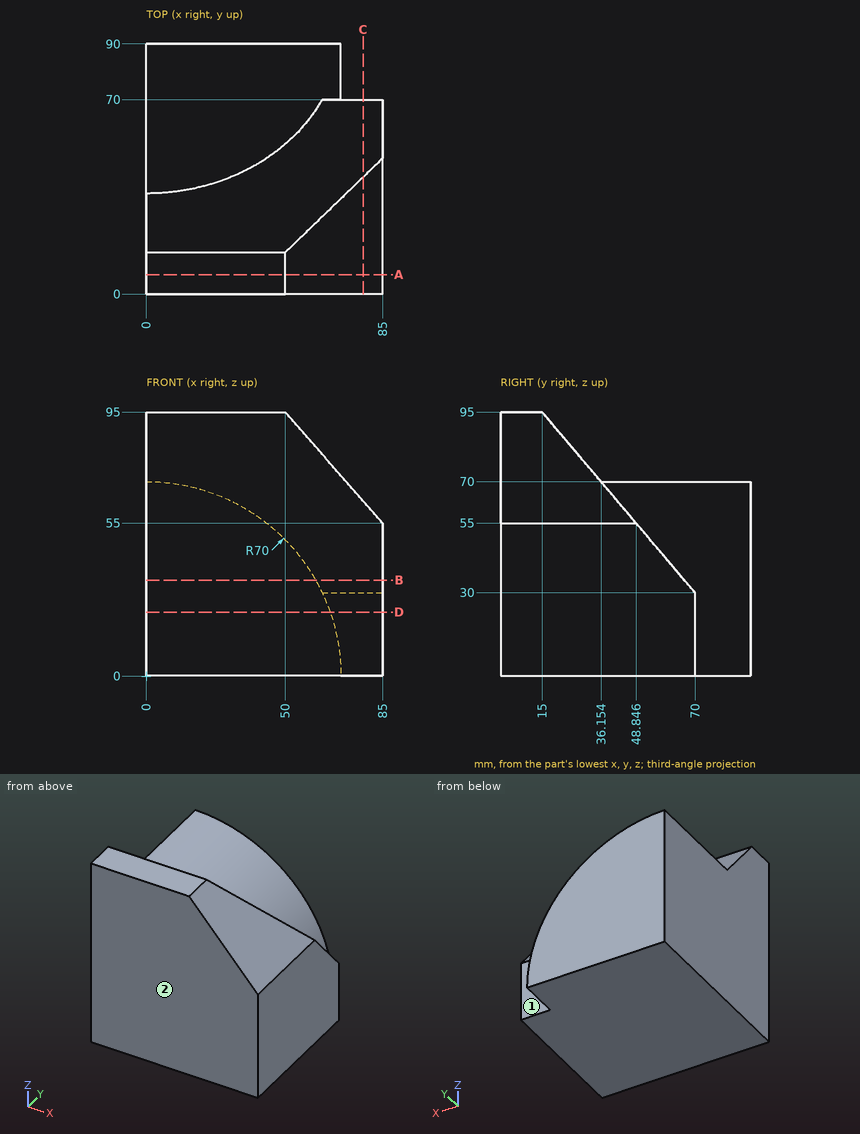
Geometry: see drawing. Coordinates: mm, zero at the bounding-box minimum. A direction names the side the tool comes from. Give positions to 0.01 mm unless a question says otherwise; leave off trailing zeros. Order: outer loops, then holes, each group sorted by start corner. A loop starts at its lowest first (then second) coordinate and runs counter-clockwise, first axis right, second up.
Q1. Section C-C on x = 78. Output: boundary loops of the cut face in (y, z).
Checked values:
outline: (0, 0) - (70, 0) - (70, 30) - (42.08, 63) - (0, 63) - close
Q2. Set-up query: the marked faces 1 and 2. Return all of +Z, -Z, +X, -X, +Y, -Y with unobstructed straight access to the full face (end or side cutting, diameter ignored); none if empty.
Checked values:
face 1: +Z, +X, +Y
face 2: +Z, -Z, +X, -X, -Y
Q3. Section A-A on y = 7. Output: boundary loops of the cut face in (x, z).
Checked values:
outline: (0, 0) - (85, 0) - (85, 55) - (50, 95) - (0, 95) - close
Q4. Section B-B on z = 34.5. Output: boundary loops of the cut face in (x, y).
Checked values:
outline: (0, 0) - (85, 0) - (85, 66.19) - (60.91, 66.19) - (60.91, 90) - (0, 90) - close
Q5. Section D-D on z = 23. Output: boundary loops of the cut face in (x, y), and give its area (3 significant figures).
Checked values:
outline: (0, 0) - (85, 0) - (85, 70) - (66.11, 70) - (66.11, 90) - (0, 90) - close
area: 7,270 mm2
Q6. Contact query for flat-ended pins moving along their axis: pin 1 Ø1 at (x, z) = (69.5, 26) entering from +Y; pin 2 Ø1 at (x, y) = (59.5, 64.5) entering from +Z; pin 3 Ø12 at (y, z) = (77.5, 25.5) entering from +X. Output: stop coordinate, or through.
Checked values:
pin 1: stops at y = 70
pin 2: stops at z = 37.67
pin 3: stops at x = 67.23
Q7. Ray query, probe 1 along Z at (x, y) = (50, 17); probe 2 along Y at (x, z) = (77, 42.5); probe 3 along Z at (x, y) = (40, 54) (1 decimal). Return the intervals inside material, ascending.
Checked values:
probe 1: z = 0 to 92.64
probe 2: y = 0 to 59.42
probe 3: z = 0 to 57.4
